The listing builds one solid part. Answer for the finished solid, in the listing's coordinates (mm). A direction names the side the tool comes from. Coordinates: 2 decimals unless noted, no trailing zeros. Order: outer loops, then holes, each group sorted by start corner. A loop starts at its lowest first (then second) coordinate and runs counter-clockwise, first axis right, second up. Notation, with made-up numbers: (-22.75, 89.5) -> (-7.75, 89.5) arc R14 cw to (-7.75, 95.5) -> close; hole circle Ø1 at (-13, 2). An arc over 180 degrees is marked (long way). Put each result on its own line as item: value. Start each with the question number.
```python
from build123d import *

# Parameters (mm, degrees)
SKETCH1_R           = 1.625
BOSS_EXTRUDE1_DEPTH = 5
FILLET1_R           = 4
FILLET3_R           = 1.5
BOSS_EXTRUDE2_DEPTH = 3


with BuildPart() as part:
    # Sketch1 → Boss-Extrude1 (new body)
    with BuildSketch(Plane(origin=(0, 0, 0), x_dir=(1, 0, 0), z_dir=(0, 1, 0))):
        Polygon((0, 0), (5.5, 0), (5.5, 3), (12.5, 3), (12.5, 0), (18, 0), (18, 11), (9, 11), (9, 19), (18, 19), (18, 27), (0, 27), align=None)
        with Locations(Location((4, 23, 0), (0, 0, 270))):
            Circle(SKETCH1_R, mode=Mode.SUBTRACT)
        with Locations(Location((14, 23, 0), (0, 0, 270))):
            Circle(SKETCH1_R, mode=Mode.SUBTRACT)
        with Locations(Location((14, 7, 0), (0, 0, 270))):
            Circle(SKETCH1_R, mode=Mode.SUBTRACT)
        with Locations(Location((4, 7, 0), (0, 0, 270))):
            Circle(SKETCH1_R, mode=Mode.SUBTRACT)
    extrude(amount=BOSS_EXTRUDE1_DEPTH)

    # Fillet1
    fillet1_edges = [part.edges().sort_by_distance(p)[0] for p in [
        (9, 2.5, -11),
        (9, 2.5, -19),
        (18, 2.5, -11),
        (0, 2.5, -27),
        (18, 2.5, -27),
        (18, 2.5, -19),
    ]]
    fillet(fillet1_edges, radius=FILLET1_R - 0.0001)  # a hair under: the kernel refuses the full size

    # Fillet3
    fillet3_edges = [part.edges().sort_by_distance(p)[0] for p in [
        (12.5, 2.5, -3),
        (18, 2.5, 0),
        (12.5, 2.5, 0),
        (5.5, 2.5, -3),
        (5.5, 2.5, 0),
        (0, 2.5, 0),
    ]]
    fillet(fillet3_edges, radius=FILLET3_R - 0.0001)  # a hair under: the kernel refuses the full size

    # Sketch3 → Boss-Extrude2 (add)
    with BuildSketch(Plane.XY.offset(-3)):
        with BuildLine():
            Line((8.25, 0.91886117), (8.25, 0))
            Line((8.25, 0), (9.75, 0))
            Line((9.75, 0), (9.75, 0.91886117))
            ThreePointArc((9.75, 0.91886117), (9, 4.25), (8.25, 0.91886117))
        make_face()
    extrude(amount=BOSS_EXTRUDE2_DEPTH)


solid = part.part
```
(1) The part is cut by section D-D on z = -12.5. Determine the outline of the cut face in (x, y), plus the area to 3 significant figures.
(2) The part is cut by section A-A on y = 4.55. Count the separate pieces of the cut face and the enclosed holes in it, plus the area to 3 significant figures.
(3) Find the intervals of material crossed by L1, parallel to X at y = 1.5, z = -23 (3 decimals); L2, parallel to X at y = 4.25, z = -7.5; L3, parallel to Z at x = 15, y = 3.5, in increasing order.
(4) A tool of negligible diameter and unlimited length cuts with its end or side. For faces 1 (the cylindrical face through (12.05, 2.54, -2.57)), 2 (the cylindrical face through (16.859, 2.535, -9.797)), 3 (the cylindrical face through (5.098, 2.465, -8.198)), from which of +Z, -Z, +X, -X, +Y, -Y can it reach the whole face along a straight path? Write none if from no direction.
(5) This flat-tipped pin is pushed along its axis until it touches: P1, Ø0.5, axis at x = 13.5, y = 3, coming from the +Z side. Where does it stop, or does it pass through?
(6) The part is cut by section B-B on z = -2.25. Determine the outline of the cut face in (x, y), plus the area to 3 significant figures.
(7) For a pull along Z with two mould halves and no side action, classify faces 4 (the cylindrical face through (10.203, 2.535, -17.859)), 5 (the flat face through (9.75, 0.5, -1.5)), 6 (the flat face through (15, 2, 0)) as released by +Z, released by -Z, zero draft, split by the parting line, or undercut.
Worked out:
1. outline: (0, 0) -> (9.88, 0) -> (9.88, 5) -> (0, 5) -> close
1. area: 49.4 mm2
2. separate pieces: 1
2. enclosed holes: 4
2. area: 352 mm2
3. L1: 0 to 2.375, 5.625 to 12.375, 15.625 to 18
3. L2: 0 to 2.45, 5.55 to 12.45, 15.55 to 17.97
3. L3: -26.87 to -24.28, -21.72 to -19.13, -10.87 to -8.28, -5.72 to 0
4. face 1: +Z, +Y, -Y
4. face 2: +X, +Y, -Y
4. face 3: +Y, -Y
5. P1: z = -0.02
6. outline: (0, 0) -> (5.7, 0) -> (5.7, 5) -> (0, 5) -> close; (8.25, 0) -> (9.75, 0) -> (9.75, 0.92) arc R1.75 ccw (long way) to (8.25, 0.92) -> close; (12.3, 0) -> (18, 0) -> (18, 5) -> (12.3, 5) -> close
6. area: 67.8 mm2
7. face 4: undercut
7. face 5: zero draft
7. face 6: released by +Z
